Study the drawing (mm; zero at the part's minimum x, y, z) and answer. A direction names the side the tool comes from. Give positions to 0.01 mm unless a question says otherwise; leave off trailing zeros. Loops run counter-clockwise (first coordinate to the right, second up) from the corner with the lowest first, then second, coordinate; pieces in that order, holes last. Notation, with made-up numbers: (45.5, 83) - (74.5, 83) arc R30 ccw to (74.5, 107) - close; hole circle Ø8 at (30.5, 85.5). An arc over 180 degrees is marked (long way). Answer in a Markdown table with one row per item. Add a question column.
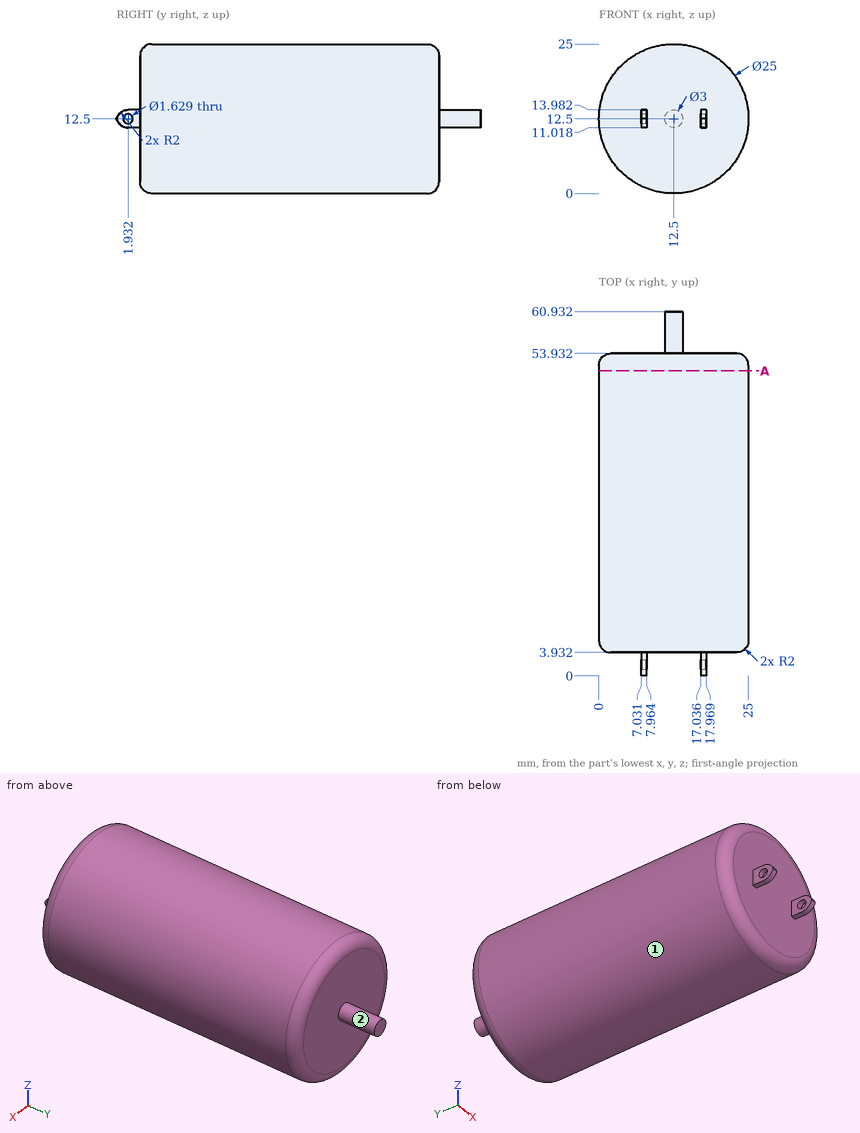
(1) A tool of negligible diameter and unlimited length cuts with its end or side. For the marked faces 1 and 2, from which of +Z, -Z, +X, -X, +Y, -Y can it reach the whole face along a straight path? Write none if from no direction.
(2) Find the intervals of material crossed by line 1 along X through (y, z) = (29, 12.75); line 2 along Y through (x, z) = (14, 4.75); line 3 along Y through (x, z) = (17.75, 13) (1 decimal), in increasing order. Write a range as [from, to].
(3) A cutting plane is placed at A-A on y = 51. Determine the outline of the cut face in (x, z).
(4) Given pin 1 Ø5 at (y, z) = (28.5, 8.5) entering from -X; pin 2 Ø4 at (y, z) = (36, 15) entering from -X; pin 3 Ø8 at (x, z) = (18.5, 19.5) entering from +Y, each flat-ended and moving along its own axis, determine where each tip first touches the part or whether it passes through.
Evaluation:
| question | item | result |
|---|---|---|
| 1 | face 1 | +Y, -Y |
| 1 | face 2 | +Y |
| 2 | line 1 | x = [0, 25] |
| 2 | line 2 | y = [3.93, 53.93] |
| 2 | line 3 | y = [0.2, 1.3], [2.6, 53.9] |
| 3 | outline | circle Ø25 at (12.5, 12.5) |
| 4 | pin 1 | stops at x = 0.09 |
| 4 | pin 2 | stops at x = 0.01 |
| 4 | pin 3 | stops at y = 53.93 |
